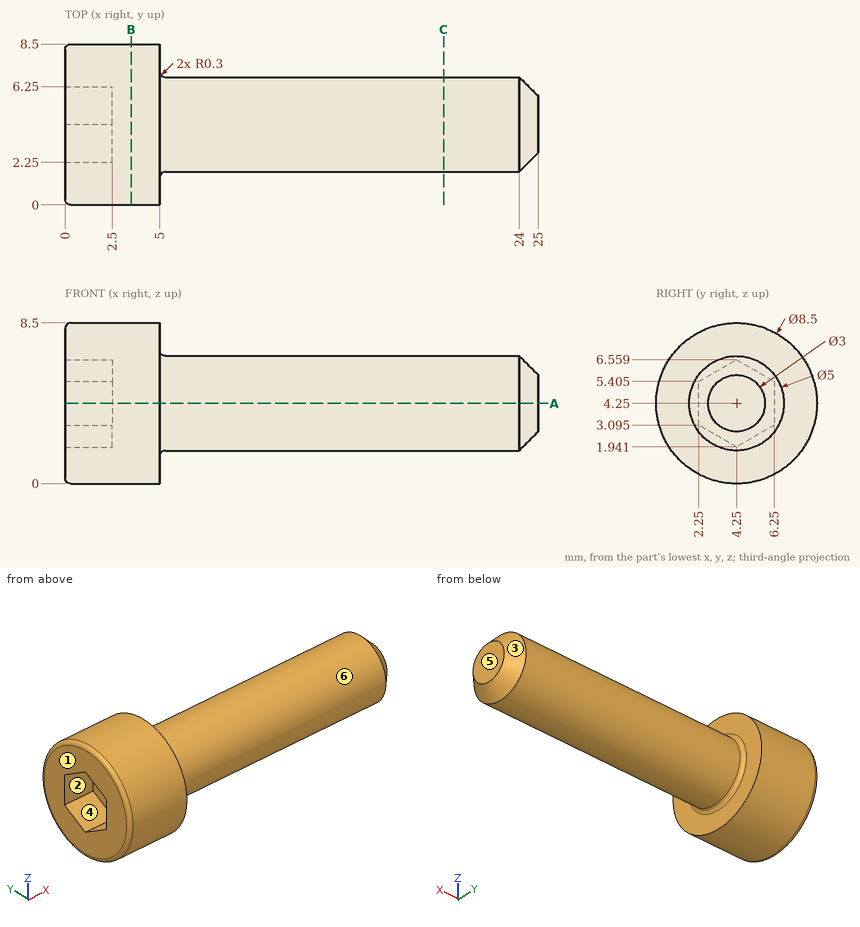
Input: dimensioned drawing with shaded views. Units: mm. Origin: part minimum x, y, z. A direction names the side the tool comes from. Round coordinates to 2 decimals unless told otherwise and drop trailing zeros. Loops run counter-clockwise (first coordinate to the right, second up) from the corner with the lowest first, then second, coordinate; pieces in that order, holes last. Notation, with made-up numbers: (42.25, 40.25) -> (83.25, 40.25) arc R29 cw to (83.25, 75.25) -> close; hole circle Ø1 at (52.5, 88). An arc over 180 degrees is marked (long way). Answer as a JSON object with one key per item and string values. Group by question number.
Q1. Section query B-B (x = 3.5). Output: boundary loops of the cut face in (y, z).
Q2. Ray query, line 1 (X direction, y = 4.75, z = 1.5); line 2 (Z direction, x = 15, y = 6.25); line 3 (Y direction, x = 14.25, z = 4.25). Return the intervals inside material, ascending. Write a range as from..to.
Q3. Section query C-C (x = 20). Output: boundary loops of the cut face in (y, z).
Q4. Contact query for flat-ended pins moving along their axis: P1, Ø0.7, axis at x = 2, z = 4, coming from the -Y side; P2, Ø1.5, axis at x = 13, z = 6.5, coming from the -Y side; P3, Ø1, axis at x = 21.5, z = 1.5, coming from the -Y side; P4, Ø1, axis at y = 2, z = 7.5, coming from the +X side. Output: stop coordinate, or through.
Q5. Access query for the marked faces 4, 5 and 6. Directions: +Z, -Z, +X, -X, +Y, -Y. A direction counts if a zero-diameter tool reaches every point of the face in a straight line with its end or side. Return the directions, or none.
Q6. Mould query, pull axis Z, two halves, no side actions, for the marked faces 1, 2 and 3. Classes: pulls with the +Z half, pulls with the -Z half, needs draft (parallel to the pull), parting line crosses it, or undercut.
Q7. Section query A-A (z = 4.25). Output: boundary loops of the cut face in (x, y).
Completed:
{
 "1": {"outline": "circle Ø8.5 at (4.25, 4.25)"},
 "2": {"line 1": "0..5", "line 2": "2.75..5.75", "line 3": "1.75..6.75"},
 "3": {"outline": "circle Ø5 at (4.25, 4.25)"},
 "4": {"P1": "y = 0", "P2": "y = 2.25", "P3": "y = 3.16", "P4": "x = 5"},
 "5": {"face 4": "-X", "face 5": "+Z, -Z, +X, +Y, -Y", "face 6": "+X"},
 "6": {"face 1": "needs draft", "face 2": "undercut", "face 3": "parting line crosses it"},
 "7": {"outline": "(0, 0.3) arc R0.3 ccw to (0.3, 0) -> (5, 0) -> (5, 1.45) arc R0.3 cw to (5.3, 1.75) -> (24, 1.75) -> (25, 2.75) -> (25, 5.75) -> (24, 6.75) -> (5.3, 6.75) arc R0.3 cw to (5, 7.05) -> (5, 8.5) -> (0.3, 8.5) arc R0.3 ccw to (0, 8.2) -> (0, 6.25) -> (2.5, 6.25) -> (2.5, 2.25) -> (0, 2.25) -> close"}
}
